```python
from build123d import *

# Parameters (mm, degrees)
SKETCH1_W           = 10.16
SKETCH1_H           = 8.255
BOSS_EXTRUDE1_DEPTH = 55.88
SKETCH2_R           = 3.7465
BOSS_EXTRUDE2_DEPTH = 12.7
SKETCH3_R           = 1.27
CUT_EXTRUDE2_DEPTH  = 70.451265332
LPATTERN1_COUNT     = 4
LPATTERN1_PITCH     = 5.08
FILLET1_R           = 1.905


with BuildPart() as part:
    # Sketch1 → Boss-Extrude1 (new body)
    with BuildSketch(Plane(origin=(0, 0, 0), x_dir=(1, 0, 0), z_dir=(0, 1, 0))):
        Rectangle(SKETCH1_W, SKETCH1_H)
    extrude(amount=BOSS_EXTRUDE1_DEPTH)

    # Sketch2 → Boss-Extrude2 (add)
    with BuildSketch(Plane(origin=(0, 55.88, 0), x_dir=(1, 0, 0), z_dir=(0, 1, 0))):
        with Locations(Location((0, 0, 0), (0, 0, 270))):
            Circle(SKETCH2_R)
    extrude(amount=BOSS_EXTRUDE2_DEPTH)

    # Sketch3 → Cut-Extrude2 (cut, through all)
    with BuildSketch(Plane(origin=(5.08, 0, 0), x_dir=(0, 0, -1), z_dir=(1, 0, 0))):
        with Locations((0, 5.08)):
            Circle(SKETCH3_R)
    cut_extrude2 = extrude(amount=-CUT_EXTRUDE2_DEPTH, mode=Mode.SUBTRACT)

    # LPattern1: Cut-Extrude2 ×4
    with Locations(*[(0, i * LPATTERN1_PITCH, 0) for i in range(1, LPATTERN1_COUNT)]):
        add(cut_extrude2, mode=Mode.SUBTRACT)

    # Fillet1
    fillet1_edges = [part.edges().sort_by_distance(p)[0] for p in [
        (0, 68.58, -3.7465),
    ]]
    fillet(fillet1_edges, radius=FILLET1_R)


solid = part.part
```
The listing builds one solid part. Answer for the finished solid, in the listing's coordinates (mm). A direction names the side the tool comes from. Coordinates: 2 decimals unless noted, no trailing zeros. Write each loop counter-clockwise with the first axis right and the second up, starting at its lowest first coordinate (ties: lowest second). Pieces come first, ordered by that corner, then holes. Notation, with made-up numbers: M -33.5,63 L -10.5,63 A24 cw -10.5,91 Z; hole C 78,-29 d6. An arc over 180 degrees is marked long. Use a Markdown table: item, result. Add a question column.
1. Straight lines are drawn through the part: line 1 along Y through (x, z) = (-1.5, 0); line 2 along Y through (x, z) = (-3, 0); line 3 along Y through (x, z) = (3.25, 3.5). For each, find the intervals that lie inside material, in ascending order. Write a range as [from, to].
2. Which of the six approach directions +Z, -Z, +X, -X, +Y, -Y give full straight-line access (tool end or side, diameter ignored) to faces 5 (the flat face through (-1.2, 55.88, -3.73)), 6 (the flat face through (0, 0, 0))?
3. Given P1, Ø2, axis at y = 10.16, z = 0, coming from the +X side, flat-ended and moving along its own axis, determine where the tip first touches the part or whether it passes through.
4. For a pull along Z with two mould halves and no side action, classify faces 1 (the flat face through (-5.08, 28, 0)), 2 (the cylindrical face through (-1.435, 61.202, 3.461)), 3 (the cylindrical face through (0.07, 21.58, 0.17)), 4 (the cylindrical face through (0.07, 16.5, 0.17)) as +Z half, -Z half, draft (parallel to the pull), parting line (faces both ways), or undercut.
5. Section A-A (y = 15.24) is taken. Give the vertices of the cut face in (x, z), plus the area to 3 significant figures.
6. Section B-B (x = 2.5) is taken. Count the separate pieces of the cut face and the enclosed holes in it, plus the area to 3 significant figures.
Data:
| question | item | result |
|---|---|---|
| 1 | line 1 | y = [0, 3.81], [6.35, 8.89], [11.43, 13.97], [16.51, 19.05], [21.59, 68.58] |
| 1 | line 2 | y = [0, 3.81], [6.35, 8.89], [11.43, 13.97], [16.51, 19.05], [21.59, 68.19] |
| 1 | line 3 | y = [0, 55.88] |
| 2 | face 5 | +Y |
| 2 | face 6 | +Z, -Z, +X, -X, -Y |
| 3 | P1 | passes through |
| 4 | face 1 | draft |
| 4 | face 2 | parting line |
| 4 | face 3 | undercut |
| 4 | face 4 | undercut |
| 5 | outline | M -5.08,-4.13 L 5.08,-4.13 L 5.08,-1.27 L -5.08,-1.27 Z; M -5.08,1.27 L 5.08,1.27 L 5.08,4.13 L -5.08,4.13 Z |
| 5 | area | 58.1 mm2 |
| 6 | separate pieces | 1 |
| 6 | enclosed holes | 4 |
| 6 | area | 509 mm2 |
